from build123d import *

# Parameters (mm, degrees)
SM_BASE_FLANGE_1_DEPTH            = 2
SKETCH_6_R                        = 7.6
SKETCH_6_R_2                      = 1.65
CUT_EXTRUDE_1_DEPTH               = 10
SM_EDGE_FLANGE_1_STRIP_W          = 9.4732
SM_EDGE_FLANGE_1_STRIP_H          = 2
SM_EDGE_FLANGE_1_STRIP_CUT_DEPTH  = 22.74
SM_EDGE_FLANGE_1_RELIEF_W         = 10.4732
SM_EDGE_FLANGE_1_RELIEF_H         = 1
SM_EDGE_FLANGE_1_RELIEF_CUT_DEPTH = 2
SM_EDGE_FLANGE_1_DEPTH            = 22.74
CUT_EXTRUDE_2_DEPTH               = 10
FILLET_1_R                        = 4
CUT_EXTRUDE_3_DEPTH               = 10
FILLET_2_R                        = 1
FILLET_3_R                        = 13


# Sheet-metal steps are written as plain solids
with BuildPart() as part:
    # Sketch 1 → 基体-法兰1 (new body)
    with BuildSketch(Plane.XY):
        Polygon((0, 0), (0, -7.5), (42.435244785, -32), (80, -32), (80, -12), (59.215390309, 0), align=None)
    extrude(amount=-SM_BASE_FLANGE_1_DEPTH)

    # 草图6 → 切除-拉伸1 (cut)
    with BuildSketch(Plane.XY):
        with Locations((58.5, -16.7)):
            Circle(SKETCH_6_R)
        with Locations((73.5, -16.7)):
            Circle(SKETCH_6_R_2)
        with Locations((43.5, -16.7)):
            Circle(SKETCH_6_R_2)
    extrude(amount=-CUT_EXTRUDE_1_DEPTH, mode=Mode.SUBTRACT)

    # 边线-法兰1 strip (across the edge) → 边线-法兰1 strip cut (cut)
    with BuildSketch(Plane(origin=(22.74, 0, 0), x_dir=(0, -1, 0), z_dir=(-1, 0, 0))):
        with Locations((-4, -1)):
            Rectangle(SM_EDGE_FLANGE_1_STRIP_W, SM_EDGE_FLANGE_1_STRIP_H)
    extrude(amount=SM_EDGE_FLANGE_1_STRIP_CUT_DEPTH, mode=Mode.SUBTRACT)

    # 边线-法兰1 relief (on the sheet) → 边线-法兰1 relief cut (cut)
    with BuildSketch(Plane(origin=(22.74, -0.7366, 0), x_dir=(0, -1, 0), z_dir=(0, 0, 1))):
        with Locations((-4.2366, 0.5)):
            Rectangle(SM_EDGE_FLANGE_1_RELIEF_W, SM_EDGE_FLANGE_1_RELIEF_H)
    extrude(amount=-SM_EDGE_FLANGE_1_RELIEF_CUT_DEPTH, mode=Mode.SUBTRACT)

    # 边线-法兰1 section (across the edge) → 边线-法兰1 (add)
    with BuildSketch(Plane(origin=(22.74, 0, 0), x_dir=(0, -1, 0), z_dir=(-1, 0, 0))):
        with BuildLine():
            Line((-2, 0.7366), (-2, 32))
            Line((-2, 32), (0, 32))
            Line((0, 32), (0, 0.7366))
            ThreePointArc((0, 0.7366), (0.215745145, 0.215745145), (0.7366, 0))
            Line((0.7366, 0), (0.7366, -2))
            ThreePointArc((0.7366, -2), (-1.198468417, -1.198468417), (-2, 0.7366))
        make_face()
    extrude(amount=SM_EDGE_FLANGE_1_DEPTH)

    # 草图12 → 切除-拉伸2 (cut)
    with BuildSketch(Plane(origin=(0, 2, 0), x_dir=(1, 0, 0), z_dir=(0, 1, 0))):
        with BuildLine():
            Line((10.49, -26.75), (10.49, -21.25))
            ThreePointArc((10.49, -21.25), (12.74, -19), (14.99, -21.25))
            Line((14.99, -21.25), (14.99, -26.75))
            ThreePointArc((14.99, -26.75), (12.74, -29), (10.49, -26.75))
        make_face()
        with BuildLine():
            Line((10.49, -12.25), (10.49, -6.75))
            ThreePointArc((10.49, -6.75), (12.74, -4.5), (14.99, -6.75))
            Line((14.99, -6.75), (14.99, -12.25))
            ThreePointArc((14.99, -12.25), (12.74, -14.5), (10.49, -12.25))
        make_face()
    extrude(amount=-CUT_EXTRUDE_2_DEPTH, mode=Mode.SUBTRACT)

    # 圆角1
    fillet_1_edges = [part.edges().sort_by_distance(p)[0] for p in [
        (59.215390309, 0, -1),
        (80, -12, -1),
        (42.435244785, -32, -1),
        (0, -7.5, -1),
        (22.74, 1, 32),
        (0, 1, 32),
    ]]
    fillet(fillet_1_edges, radius=FILLET_1_R)

    # 草图14 → 切除-拉伸3 (cut)
    with BuildSketch(Plane(origin=(0, 0, -2), x_dir=(-1, 0, 0), z_dir=(0, 0, -1))):
        Polygon((-36.859263982, -19.274986727), (-27.659263982, -16.364230162), (-26.84, -7), (-41.14, -7), align=None)
    extrude(amount=-CUT_EXTRUDE_3_DEPTH, mode=Mode.SUBTRACT)

    # 圆角2
    fillet_2_edges = [part.edges().sort_by_distance(p)[0] for p in [
        (26.84, -7, -1),
        (27.659263982, -16.364230162, -1),
        (36.859263982, -19.274986727, -1),
        (41.14, -7, -1),
    ]]
    fillet(fillet_2_edges, radius=FILLET_2_R)

    # 圆角3
    fillet_3_edges = [part.edges().sort_by_distance(p)[0] for p in [
        (80, -32, -1),
    ]]
    fillet(fillet_3_edges, radius=FILLET_3_R)


solid = part.part
Geometry: final body of the model. Coordinates: model frame, mm. A direction names the side the tool comes from. Round coordinates to 2 decimals unless told otherwise and drop trailing zeros. Order: outer loops, then holes, each group sorted by start corner. A loop starts at its lowest first (then second) coordinate and runs counter-clockwise, first axis right, second up.
Q1. Mould query, pull axis Z, two halves, no side actions, for faces 1 (the face through (39, -16, 0)), 2 (the face through (79.449, -12.284, -1.014)), 3 (the face through (12.7, 1, 4.5)), 4 (the face through (14.99, 1, 9)). Classes: released by +Z, released by -Z, zero draft, split by the parting line, or undercut.
Result sheet:
face 1: released by +Z
face 2: zero draft
face 3: undercut
face 4: undercut
Q2. Pin query (flat end, axial travel): pin 1 (6 mm diameter, centred on x = 9, z = 26, fed in from -Y); pin 2 (5.5 mm diameter, centred on x = 43.5, y = -16.7, fed in from +Z); pin 3 (1 mm diameter, centred on x = 31, z = -1.5, fed in from -Y). Return the tip coordinate at first contact, or that it passes through.
Result sheet:
pin 1: stops at y = 0
pin 2: stops at z = 0
pin 3: stops at y = -25.69
Q3. Access query for faces 5 (the face through (23.74, -1, -1)), 6 (the face through (11, 1, 32)), 7 (the face through (12, 2, 16)), 8 (the face through (12.8, 1, 29)), 9 (the face through (32.2, -17.8, -1)). Directions: +Z, -Z, +X, -X, +Y, -Y. A direction counts if a zero-diameter tool reaches every point of the face in a straight line with its end or side. Return the directions, or none.
Result sheet:
face 5: +Z, -Z, +Y
face 6: +Z, +X, -X, +Y, -Y
face 7: +Z, -Z, +X, -X, +Y
face 8: +Y, -Y
face 9: +Z, -Z
Q4. Section B-B, the plane y = -13.5. Output: boundary loops of the cut face in (x, z).
Result sheet:
outline: (10.39, -2) - (27.41, -2) - (27.41, 0) - (10.39, 0) - close; (38.87, -2) - (51.61, -2) - (51.61, 0) - (38.87, 0) - close; (65.39, -2) - (79.92, -2) - (79.92, 0) - (65.39, 0) - close
Q5. Section A-A, the plane x = 55. Output: boundary loops of the cut face in (y, z).
Result sheet:
outline: (-32, -2) - (-23.45, -2) - (-23.45, 0) - (-32, 0) - close; (-9.95, -2) - (0, -2) - (0, 0) - (-9.95, 0) - close
Q6. Material intervals for probe 1 along X at (y, z) = (-16, -1); probe 2 along Y at (x, z) = (58.5, -0.9); probe 3 along Z at (x, y) = (52, -26), sorted ascending.
Result sheet:
probe 1: x = 14.72 to 27.68, 38 to 42.01, 44.99 to 50.93, 66.07 to 72.01, 74.99 to 80
probe 2: y = -32 to -24.3, -9.1 to -0.02
probe 3: z = -2 to 0
Q7. Section D-D, the plane z = 2.5. Output: boundary loops of the cut face in (x, y).
Result sheet:
outline: (0, 0) - (22.74, 0) - (22.74, 2) - (0, 2) - close
Q8. Section C-C, the plane y = -23. Output: boundary loops of the cut face in (x, z).
Result sheet:
outline: (26.85, -2) - (54.25, -2) - (54.25, 0) - (26.85, 0) - close; (62.75, -2) - (79.37, -2) - (79.37, 0) - (62.75, 0) - close
